```python
from build123d import *

# Parameters (mm, degrees)
CROQUIS1_R              = 10
SALIENTE_EXTRUIR1_DEPTH = 10
CROQUIS2_R              = 15
CROQUIS2_R_2            = 10
SALIENTE_EXTRUIR2_DEPTH = 40
CROQUIS3_W              = 30
CROQUIS3_H              = 30
SALIENTE_EXTRUIR3_DEPTH = 10
BOSS_EXTRUDE1_START     = 15
SKETCH1_R               = 15
SKETCH1_R_2             = 10
BOSS_EXTRUDE1_DEPTH     = 15


with BuildPart() as part:
    # Croquis1 → Saliente-Extruir1 (new body)
    with BuildSketch(Plane.XY):
        with BuildLine():
            Line((-44.292513238, 22.5), (85.707486762, 22.5))
            ThreePointArc((85.707486762, 22.5), (100.707486762, 7.5), (85.707486762, -7.5))
            Line((85.707486762, -7.5), (-44.292513238, -7.5))
            ThreePointArc((-44.292513238, -7.5), (-59.292513238, 7.5), (-44.292513238, 22.5))
        make_face()
        with Locations((-44.292513238, 7.5)):
            Circle(CROQUIS1_R, mode=Mode.SUBTRACT)
        with Locations(Location((85.707486762, 7.5, 0), (0, 0, 180))):
            Circle(CROQUIS1_R, mode=Mode.SUBTRACT)
    extrude(amount=SALIENTE_EXTRUIR1_DEPTH)

    # Croquis2 → Saliente-Extruir2 (add)
    with BuildSketch(Plane.XY.offset(10)):
        with Locations(Location((-44.292513238, 7.5, 0), (0, 0, 270))):
            Circle(CROQUIS2_R)
        with Locations((-44.292513238, 7.5)):
            Circle(CROQUIS2_R_2, mode=Mode.SUBTRACT)
    extrude(amount=SALIENTE_EXTRUIR2_DEPTH)

    # Croquis3 → Saliente-Extruir3 (add)
    with BuildSketch(Plane.XY.offset(50)):
        with Locations((-44.292513238, 7.5)):
            Rectangle(CROQUIS3_W, CROQUIS3_H)
    extrude(amount=SALIENTE_EXTRUIR3_DEPTH)

    # Sketch1 → Boss-Extrude1 (add)
    with BuildSketch(Plane(origin=(0, 0, 0), x_dir=(-1, 0, 0), z_dir=(0, 0, -1)).offset(BOSS_EXTRUDE1_START)):
        with Locations((44.292513238, 7.5)):
            Circle(SKETCH1_R)
        with Locations((44.292513238, 7.5)):
            Circle(SKETCH1_R_2, mode=Mode.SUBTRACT)
    extrude(amount=-BOSS_EXTRUDE1_DEPTH)


solid = part.part
```
Geometry check sheet. Reference: the model listing, model coordinates, mm. A direction names the side the tool comes from. Give positions to 0.01 mm unless a question says otherwise; leave off trailing zeros. Order: outer loops, then holes, each group sorted by start corner. A loop starts at its lowest first (then second) coordinate and runs counter-clockwise, first axis right, second up. Notation, with made-up numbers: (12.25, -30.75) - (67.25, -30.75) arc R27 ccw to (67.25, 3.25) - close; hole circle Ø5 at (-24.5, 39.5). An arc over 180 degrees is marked (long way). Answer in a Markdown table with one row per item. Add a question column.
Q1. Cross-section at C-C, the plane z = 12. Enter the section's corners in (x, y).
Q2. Cross-section at B-B, the plane x = 65.5. Enter the section's corners in (y, z).
Q3. Tool access check on faces 1 (the flat face through (-56, -4, 50)), 2 (the flat face through (-32, -4, 50)), 3 (the flat face through (-33, 19, 50)). Record the directions out of +Z, -Z, +X, -X, +Y, -Y that give a thin tool (end or side, any length) a straight path to the whole face; none if there is none.
Q4. Cross-section at D-D, the plane y = 9.5. Enter the section's corners in (x, z), then the cut area to 3 significant figures.
Q5. Mould release check, pull along Y, two halves, no side actions. Record for faces 4 (the flat face through (-45, -7.5, 55)), 5 (the flat face through (-54, 4, -15)), 6 (the cylindrical face through (93.078, 0.742, 4.93)): pulls with the +Y half, pulls with the -Y half, needs draft (parallel to the pull), parting line crosses it, or undercut.
Q6. Gauge pin test, flat ends, axial feed: pin 1 (16 mm diameter, centred on x = -44.29, y = 7.5, fed in from -Z); pin 2 (2 mm diameter, centred on x = -29, y = 0.5, fed in from -Z); pin 3 (5 mm diameter, centred on y = 2.5, z = 5, fed in from +X). Record the tip position at first contact, or that the pin passes through.
Q7. Material ranges on probe 1 along X at (y, z) = (7.5, -6.25); probe 2 along Z at (x, y) = (58.5, 7); probe 3 along X at (y, z) = (9.5, -6), recorded low to high. Write a range as from..to.
Q8. Cross-section at A-A, the plane y = 2. Enter the section's corners in (x, z).
Check values:
| question | item | result |
|---|---|---|
| 1 | outline | circle Ø30 at (-44.29, 7.5); hole circle Ø20 at (-44.29, 7.5) |
| 2 | outline | (-7.5, 0) - (22.5, 0) - (22.5, 10) - (-7.5, 10) - close |
| 3 | face 1 | -Z, -X, -Y |
| 3 | face 2 | +X, -Y |
| 3 | face 3 | +X, +Y |
| 4 | outline | (-59.29, 50) - (-59.16, 50) - (-59.16, -15) - (-54.09, -15) - (-54.09, 50) - (-34.49, 50) - (-34.49, -15) - (-29.43, -15) - (-29.43, 0) - (75.91, 0) - (75.91, 10) - (-29.43, 10) - (-29.43, 50) - (-29.29, 50) - (-29.29, 60) - (-59.29, 60) - close; (95.51, 0) - (100.57, 0) - (100.57, 10) - (95.51, 10) - close |
| 4 | area | 2,060 mm^2 |
| 5 | face 4 | pulls with the -Y half |
| 5 | face 5 | needs draft |
| 5 | face 6 | undercut |
| 6 | pin 1 | stops at z = 50 |
| 6 | pin 2 | stops at z = 0 |
| 6 | pin 3 | stops at x = 100.5 |
| 7 | probe 1 | x = -59.29..-54.29, -34.29..-29.29 |
| 7 | probe 2 | z = 0..10 |
| 7 | probe 3 | x = -59.16..-54.09, -34.49..-29.43 |
| 8 | outline | (-59.29, 50) - (-58.25, 50) - (-58.25, -15) - (-52.64, -15) - (-52.64, 50) - (-35.94, 50) - (-35.94, -15) - (-30.34, -15) - (-30.34, 0) - (77.36, 0) - (77.36, 10) - (-30.34, 10) - (-30.34, 50) - (-29.29, 50) - (-29.29, 60) - (-59.29, 60) - close; (94.06, 0) - (99.66, 0) - (99.66, 10) - (94.06, 10) - close |
